Autodesk Inventor part; units mm, degrees
ref_plane "YZ Plane" through (0, 0, 0) normal (1, 0, 0) x (0, 1, 0)
ref_plane "XZ Plane" through (0, 0, 0) normal (0, 1, 0) x (-1, 0, 0)
ref_plane "XY Plane" through (0, 0, 0) normal (0, 0, 1) x (1, 0, 0)
sketch "Skizze1" plane through (0, 0, 0) normal (0, 0, 1) x (1, 0, 0)
  line L0 (0, 0) -> (0, 22)
  line L1 (0, 22) -> (40, 22)
  line L2 (40, 22) -> (40, 21.5)
  line L3 (40, 21.5) -> (50, 21.5)
  line L4 (50, 21.5) -> (50, 0)
  line L5 (50, 0) -> (0, 0)
  dimension "d0" = 44
  dimension "d1" = 43
  dimension "d2" = 40
  dimension "d3" = 50
revolve "Umdrehung1" add sketch "Skizze1" angle 360 about axis through (50, 0, 0) along (-1, 0, 0)
chamfer "Fasen1" distance 2 angle 15 1 edges at (0, -22, 0) measured on face at (0, -5.3524, -1.755)
sketch "Skizze2" plane through (50, 0, 0) normal (1, 0, 0) x (0, 0, -1)
  circle A0 centre (0, 0) radius 17.5
  dimension "d8" = 35
extrude "Extrusion1" cut sketch "Skizze2" against normal up to surface (50 mm away)
properties part number "Zylinder_laufbuechse" material "Glas"
Part model, mm, in its own coordinate system. A direction names the side the tool comes from. Coordinates: 2 decimals unless noted, no trailing zeros. Order: outer loops, then holes, each group sorted by start corner. A loop starts at its lowest first (then second) coordinate and runs counter-clockwise, first axis right, second up. Notation, with made-up numbers: M -34,-22 L 8,-22 A31 cw 8,10 Z; hole C 16.5,14.5 d3. An arc over 180 degrees is marked long. One line per question, with ' | ' between items.
Q1. 3-axis set-ups, long thin cutter, end or side, ignore diameter. For faces 4 (the face through (40, 9.7, 19.5)), 5 (the face through (50, 3.1, 17.4)): which of +Z, -Z, +X, -X, +Y, -Y reach the whole face in a straight line?
A:
face 4: +X | face 5: +Z, -Z, +X, +Y, -Y
Q2. Slice it at D-D (x = 46.5). Give the cut face in (y, z), and give its area (3 significant figures).
A:
outline: C 0,0 d43; hole C 0,0 d35 | area: 490 mm^2
Q3. Two-plate mould, pull along Y, no slides. Class faces 1 (the face through (20.544, -4.769, -21.477)), 2 (the face through (0, 0, 18)), 3 (the face through (25.35, -10.648, 13.887)): +Y half, -Y half, draft (parallel to the pull), parting line (faces both ways), or undercut.
A:
face 1: parting line | face 2: draft | face 3: undercut
Q4. Drill centre lines: line 1 (Y direction, x = 35, z = 0); line 2 (Y direction, x = 16, z = 9); line 3 (Z direction, x = 32.5, y = -11). Where is each one in solid material? Low to high.
A:
line 1: y = -22 to -17.5, 17.5 to 22 | line 2: y = -20.07 to -15.01, 15.01 to 20.07 | line 3: z = -19.05 to -13.61, 13.61 to 19.05
Q5. Slice it at C-C (x = 39). Give the cut face in (y, z), and give its area (3 significant figures).
A:
outline: C 0,0 d44; hole C 0,0 d35 | area: 558 mm^2
Q6. Slice it at A-A (y = 0). Give the cut face in (x, z), and give its area (3 significant figures).
A:
outline: M 0,-20 L 0.54,-22 L 40,-22 L 40,-21.5 L 50,-21.5 L 50,-17.5 L 0,-17.5 Z; M 0,17.5 L 50,17.5 L 50,21.5 L 40,21.5 L 40,22 L 0.54,22 L 0,20 Z | area: 439 mm^2
Q7. Pin check, flat tips, straight feed: P1, Ø8, axis at x = 13.5, y = 12, coming from the -Z side; P2, Ø2, axis at y = -13, z = 6.5, coming from the -X side; P3, Ø5, axis at x = 44, y = -14.5, coming from the +Z side; P4, Ø1, axis at x = 21, z = 3, coming from the +Y side. Stop position of each tip, or through.
A:
P1: stops at z = -20.49 | P2: passes through | P3: stops at z = 17.84 | P4: stops at y = 21.86
